Check sheet for the modelled part. Datum: model origin and axes. Units: mm. Face numbers are marked on the shaded views. A direction names the side the tool comes from. Round coordinates to 2 decimals unless told otherwise and drop trailing zeros. Write each loop counter-clockwise with the first axis right and the second up, starting at its lowest first coordinate (ties: lowest second). Pieces come first, ordered by that corner, then holes.
Item 1: Set-up check for the marked faces 1 and 2: record each of +Z, -Z, +X, -X, +Y, -Y from which the full face is reachable in a straight line by a thin tool's end or side.
Item 2: Material ranges on line 1 along Y through (x, z) = (-45.5, 11); line 2 along Z through (x, y) = (-35.5, 27); line 3 along X through (y, z) = (-62.5, 88), recorded low to high.
Item 3: Depth check by flat-ended pin: pin 1 (12 mm diameter, centred on y = 44, z = 38, fed in from -X); pin 2 (6.5 mm diameter, centred on x = -9, y = 11, fed in from -Z). Enter the tip coordinate at first touch or a pass-through.
Item 4: Section check A-A, the plane y = 0. Record the cut outline in (x, z).
Item 5: Section check B-B, the plane x = -85. Record the cut outline in (y, z), plus the area to 3 significant figures.
Item 6: Section check D-D, the plane y = -186. Record the cut outline in (x, z).
Item 7: Section check C-C, the plane z = 38.5. Record the cut outline in (x, y).
from build123d import *

# Parameters (mm, degrees)
F0_W     = 152.4
F0_H     = 609.6
F1_DEPTH = 12.7
F2_W     = 12.7
F2_H     = 609.6
F3_DEPTH = 101.6
F5_DEPTH = 25
F6_R     = 25.4
F7_DEPTH = 50.8


with BuildPart() as f1:
    # F0 (on Top) → F1 (new body)
    with BuildSketch(Plane.XY):
        with Locations((-76.2, 0)):
            Rectangle(F0_W, F0_H)
    extrude(amount=F1_DEPTH)

    # F2 (on face) → F3 (join)
    with BuildSketch(Plane.XY.offset(12.7)):
        with Locations((-6.35, 0)):
            Rectangle(F2_W, F2_H)
    extrude(amount=F3_DEPTH)

    # F4 (on face) → F5 (cut)
    with BuildSketch(Plane.XY.offset(12.7)):
        with BuildLine():
            Line((-38.1, 282.4), (-127, 282.4))
            ThreePointArc((-127, 282.4), (-130, 279.4), (-127, 276.4))
            Line((-127, 276.4), (-38.1, 276.4))
            ThreePointArc((-38.1, 276.4), (-35.1, 279.4), (-38.1, 282.4))
        make_face()
        with BuildLine():
            Line((-38.1, -276.4), (-127, -276.4))
            ThreePointArc((-127, -276.4), (-130, -279.4), (-127, -282.4))
            Line((-127, -282.4), (-38.1, -282.4))
            ThreePointArc((-38.1, -282.4), (-35.1, -279.4), (-38.1, -276.4))
        make_face()
    extrude(amount=-F5_DEPTH, mode=Mode.SUBTRACT)

    # F6 (on face) → F7 (cut)
    with BuildSketch(Plane(origin=(0, 0, 0), x_dir=(1, 0, 0), z_dir=(0, 0, -1))):
        Circle(F6_R)
    extrude(amount=-F7_DEPTH, mode=Mode.SUBTRACT)


solid = f1.part
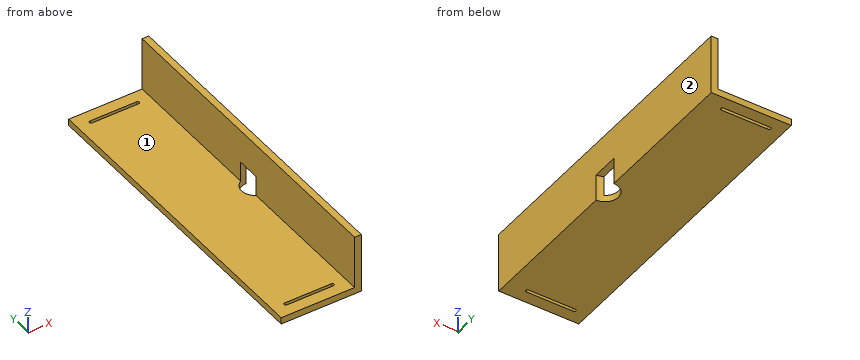
Values found:
1. face 1: +Z, -X, +Y, -Y
1. face 2: +Z, -Z, +X, +Y, -Y
2. line 1: y = -304.8 to -282.4, -276.4 to 276.4, 282.4 to 304.8
2. line 2: z = 0 to 12.7
2. line 3: x = -12.7 to 0
3. pin 1: stops at x = -12.7
3. pin 2: stops at z = 50.8
4. outline: (-152.4, 0) - (-25.4, 0) - (-25.4, 12.7) - (-152.4, 12.7) - close; (-12.7, 50.8) - (0, 50.8) - (0, 114.3) - (-12.7, 114.3) - close
5. outline: (-304.8, 0) - (-282.4, 0) - (-282.4, 12.7) - (-304.8, 12.7) - close; (-276.4, 0) - (276.4, 0) - (276.4, 12.7) - (-276.4, 12.7) - close; (282.4, 0) - (304.8, 0) - (304.8, 12.7) - (282.4, 12.7) - close
5. area: 7,590 mm2
6. outline: (-152.4, 0) - (0, 0) - (0, 114.3) - (-12.7, 114.3) - (-12.7, 12.7) - (-152.4, 12.7) - close
7. outline: (-12.7, -304.8) - (0, -304.8) - (0, -25.4) arc R25.4 cw to (-12.7, -22) - close; (-12.7, 22) arc R25.4 cw to (0, 25.4) - (0, 304.8) - (-12.7, 304.8) - close
